Source: CAD feature listing. Evaluate the final solid. Frame: model axes, mm. Face numbers are marked on the shaded views. A direction names the side the tool comes from. Round coordinates to 2 decimals unless told otherwise and drop trailing zeros. Loops run counter-clockwise (first coordinate to the right, second up) from the corner with the lowest first, then second, coordinate; pieces in that order, holes last. Notation, with made-up numbers: (-0.75, -27) -> (27.25, -27) arc R14 cw to (27.25, -2) -> close; hole circle Ø11 at (23, 11). An arc over 180 degrees is marked (long way). Put each result on its own line as item: value. Start each with the question number.
1. Draft query along X for the marked faces 1, 2 and 3. Return one class per face: pulls with the +X half, pulls with the -X half, needs draft (parallel to the pull), parting line crosses it, or undercut.
2. Cut plane C-C (x = 64.5). Return the cut outline in (y, z), then the cut area to 3 significant figures.
3. Material intervals for L1, parallel to X at y = 18.5, z = 36; L2, parallel to Y at x = 6.5, z = 26; L3, parallel to Z at x = 24.5, y = 38.5, sorted ascending.
4. Cut plane B-B (y = 31.5). Return the cut outline in (x, z), then the cut area to 3 significant figures.
5. Set-up query: the marked faces 4 and 5. Return all of +Z, -Z, +X, -X, +Y, -Y with unobstructed straight access to the full face (end or side cutting, diameter ignored); none if empty.
6. Contact query for flat-ended pins moving along their axis: pin 1 (10 mm diameter, centred on x = -32, y = -26, fed in from -Z); pin 2 (6 mm diameter, centred on x = 6, y = -29, fed in from +Z). Output: stop coordinate, or through.
7. Cut plane A-A (z = 27). Return the cut outline in (x, y), then the cut area to 3 significant figures.
```python
from build123d import *

# Parameters (mm, degrees)
F0_W     = 150
F0_H     = 100
F1_DEPTH = 40
F2_R     = 5
F3_T     = -3
F4_W     = 146
F4_H     = 96
F5_DEPTH = 2
F6_R     = 3


with BuildPart() as f1:
    # F0 (on Top) → F1 (new body)
    with BuildSketch(Plane.XY):
        Rectangle(F0_W, F0_H)
    extrude(amount=F1_DEPTH)

    # F2
    f2_edges = [f1.edges().sort_by_distance(p)[0] for p in [
        (75, 50, 20),
        (-75, 50, 20),
        (-75, -50, 20),
        (75, -50, 20),
    ]]
    fillet(f2_edges, radius=F2_R)

    # F3
    f3_openings = [f1.faces().sort_by_distance(p)[0] for p in [
        (0, 0, 40),
    ]]
    offset(amount=F3_T, openings=f3_openings)

    # F4 (on face) → F5 (cut)
    with BuildSketch(Plane.XY.offset(40)):
        Rectangle(F4_W, F4_H)
    extrude(amount=-F5_DEPTH, mode=Mode.SUBTRACT)

    # F6
    f6_edges = [f1.edges().sort_by_distance(p)[0] for p in [
        (73, 48, 39),
        (73, -48, 39),
        (-73, 48, 39),
        (-73, -48, 39),
    ]]
    fillet(f6_edges, radius=F6_R)


solid = f1.part
```
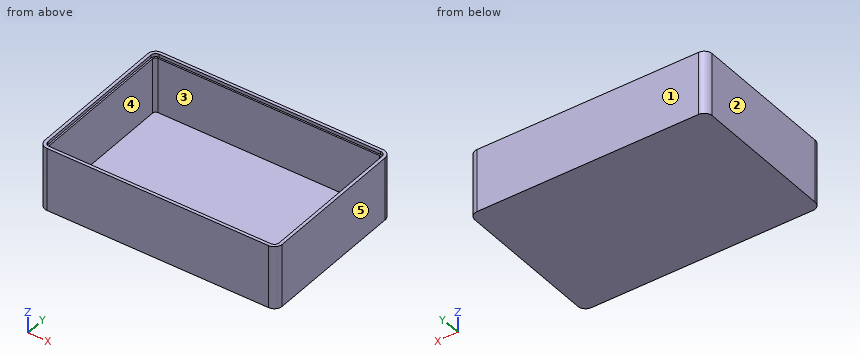
Solution:
1. face 1: needs draft
1. face 2: pulls with the -X half
1. face 3: undercut
2. outline: (-50, 0) -> (50, 0) -> (50, 40) -> (48, 40) -> (48, 38) -> (47, 38) -> (47, 3) -> (-47, 3) -> (-47, 38) -> (-48, 38) -> (-48, 40) -> (-50, 40) -> close
2. area: 518 mm^2
3. L1: x = -75 to -72, 72 to 75
3. L2: y = -50 to -47, 47 to 50
3. L3: z = 0 to 3
4. outline: (-75, 0) -> (75, 0) -> (75, 40) -> (73, 40) -> (73, 38) -> (72, 38) -> (72, 3) -> (-72, 3) -> (-72, 38) -> (-73, 38) -> (-73, 40) -> (-75, 40) -> close
4. area: 668 mm^2
5. face 4: +Z
5. face 5: +Z, -Z, +X, +Y, -Y
6. pin 1: stops at z = 0
6. pin 2: stops at z = 3
7. outline: (-75, -45) arc R5 ccw to (-70, -50) -> (70, -50) arc R5 ccw to (75, -45) -> (75, 45) arc R5 ccw to (70, 50) -> (-70, 50) arc R5 ccw to (-75, 45) -> close; hole (-72, -45) arc R2 ccw to (-70, -47) -> (70, -47) arc R2 ccw to (72, -45) -> (72, 45) arc R2 ccw to (70, 47) -> (-70, 47) arc R2 ccw to (-72, 45) -> close
7. area: 1,450 mm^2
